Read the model definition and answer for the solid it produces. Units are mm, in the model's axes. Face numbers are marked on the shaded views. A direction names the side the tool comes from. Coordinates: 2 decimals unless noted, no trailing zeros. Loops run counter-clockwise (first coordinate to the right, second up) from the corner with the lowest first, then second, coordinate; pieces in that order, holes last.
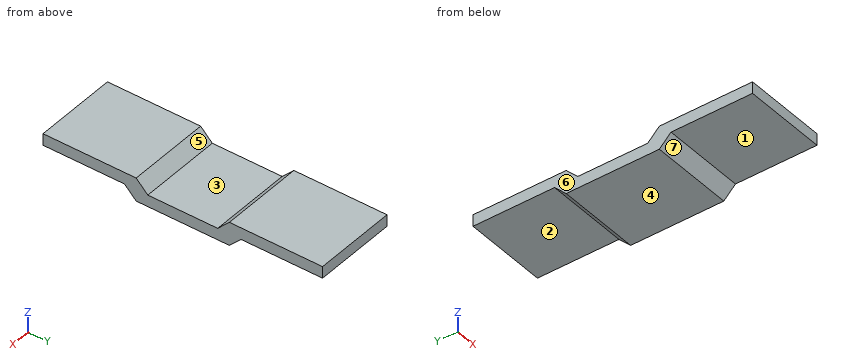
from build123d import *

# Parameters (mm, degrees)
F1_DEPTH = 11.43


with BuildPart() as f1:
    # F0 (on Right) → F1 (new body, symmetric)
    with BuildSketch(Plane.YZ):
        Polygon((-15.875, 1.5875), (-12.7, 1.5875), (-12.7, 4.7625), (-38.1, 4.7625), (-38.1, 1.5875), align=None)
        Polygon((9.525, 1.5875), (12.7, 1.5875), (12.7, 4.7625), align=None)
        Polygon((-12.7, 1.5875), (-9.525, 1.5875), (-12.7, 4.7625), align=None)
        Polygon((15.875, 1.5875), (12.7, 1.5875), (12.7, -1.5875), align=None)
        Polygon((-15.875, 1.5875), (-12.7, -1.5875), (-12.7, 1.5875), align=None)
        Polygon((12.7, 4.7625), (12.7, 1.5875), (15.875, 1.5875), (38.1, 1.5875), (38.1, 4.7625), align=None)
        Polygon((12.7, -1.5875), (12.7, 1.5875), (9.525, 1.5875), (-9.525, 1.5875), (-12.7, 1.5875), (-12.7, -1.5875), align=None)
    extrude(amount=F1_DEPTH, both=True)


solid = f1.part
Item 1: A cutting plane is placed at A-A on z = 2.5. Determine the outline of the cut face in (x, y).
Numbers:
outline: (-11.43, -38.1) - (11.43, -38.1) - (11.43, -10.44) - (-11.43, -10.44) - close; (-11.43, 10.44) - (11.43, 10.44) - (11.43, 38.1) - (-11.43, 38.1) - close
Item 2: A cutting plane is placed at D-D on z = -0.75. Determine the outline of the cut face in (x, y), then the cut area to 3 significant figures.
Numbers:
outline: (-11.43, -13.54) - (11.43, -13.54) - (11.43, 13.54) - (-11.43, 13.54) - close
area: 619 mm2
Item 3: Given pin 1 (11 mm diameter, centred on x = 5, y = 22.5, fed in from -Z); pin 2 (1 mm diameter, centred on x = 9, z = -1, fed in from +Y); pin 3 (1.5 mm diameter, centred on x = -4, z = 1.5, fed in from -Y), each flat-ended and moving along its own axis, determine where each tip first touches the part or whether it passes through.
Numbers:
pin 1: stops at z = 1.59
pin 2: stops at y = 13.79
pin 3: stops at y = -38.1
Item 4: A cutting plane is placed at B-B on x = 6.25. Determine the outline of the cut face in (y, z) (1 decimal), then the cut area to 3 significant figures.
Numbers:
outline: (-38.1, 1.6) - (-15.9, 1.6) - (-12.7, -1.6) - (12.7, -1.6) - (15.9, 1.6) - (38.1, 1.6) - (38.1, 4.8) - (12.7, 4.8) - (9.5, 1.6) - (-9.5, 1.6) - (-12.7, 4.8) - (-38.1, 4.8) - close
area: 262 mm2
Item 5: Find the intervals of material crossed by line 1 along Y through (x, z) = (-3.5, 3.5); line 2 along Z through (x, y) = (2, 30.5); line 3 along Y through (x, z) = (9.25, 2), in increasing order.
Numbers:
line 1: y = -38.1 to -11.44, 11.44 to 38.1
line 2: z = 1.59 to 4.76
line 3: y = -38.1 to -9.94, 9.94 to 38.1
Item 6: Determine the mould class of the marked faces 5, 6 and 7 for opening direction Y: released by +Y, released by -Y, zero draft, split by the parting line, or undercut.
Numbers:
face 5: undercut
face 6: zero draft
face 7: released by -Y
Item 7: A cutting plane is placed at C-C on y = 6. Determine the outline of the cut face in (x, z), then the cut area to 3 significant figures.
Numbers:
outline: (-11.43, -1.59) - (11.43, -1.59) - (11.43, 1.59) - (-11.43, 1.59) - close
area: 72.6 mm2
Item 8: Which of the six approach directions +Z, -Z, +X, -X, +Y, -Y give full straight-line access (tool end or side, diameter ignored) to the marked faces 1, 2, 3 and 4?
Numbers:
face 1: -Z, +X, -X, -Y
face 2: -Z, +X, -X, +Y
face 3: +Z, +X, -X
face 4: -Z, +X, -X, +Y, -Y
